Read the model definition and answer for the solid it produces. Units are mm, in the model's axes. A direction names the side the tool comes from. Give positions to 0.01 mm unless a question says otherwise; leave off trailing zeros. Order: outer loops, then holes, each group sorted by start corner. A loop starts at its lowest first (then second) coordinate and runs counter-clockwise, first axis right, second up.
```python
from build123d import *

# Parameters (mm, degrees)
BOSS_EXTRUDE1_DEPTH = 6.35
CUT_EXTRUDE3_DEPTH  = 4.953
SKETCH7_W           = 6.35
SKETCH7_H           = 6.35
CUT_EXTRUDE5_DEPTH  = 2.159
SKETCH9_R           = 3.175
BOSS_EXTRUDE4_DEPTH = 26.035
CUT_EXTRUDE6_REACH  = 34.945
SKETCH10_W          = 1.886216022
SKETCH10_H          = 12.7
FILLET1_R           = 1.27


with BuildPart() as part:
    # Sketch1 → Boss-Extrude1 (new body)
    with BuildSketch(Plane(origin=(0, 0, 0), x_dir=(1, 0, 0), z_dir=(0, 1, 0))):
        with BuildLine():
            Line((0.583306021, 0), (5.131693979, 0))
            ThreePointArc((5.131693979, 0), (5.661763503, 0.115908886), (6.095077487, 0.442478269))
            Line((6.095077487, 0.442478269), (9.2075, 4.953))
            Line((9.2075, 4.953), (6.0325, 4.953))
            Line((6.0325, 4.953), (6.0325, 7.112))
            Line((6.0325, 7.112), (-0.3175, 7.112))
            Line((-0.3175, 7.112), (-0.3175, 4.953))
            Line((-0.3175, 4.953), (-3.4925, 4.953))
            Line((-3.4925, 4.953), (-0.380077487, 0.442478269))
            ThreePointArc((-0.380077487, 0.442478269), (0.053236497, 0.115908886), (0.583306021, 0))
        make_face()
    extrude(amount=BOSS_EXTRUDE1_DEPTH)

    # Sketch5 → Cut-Extrude3 (cut)
    with BuildSketch(Plane.XY):
        with BuildLine():
            Line((-3.4925, 3.175), (-3.4925, 6.35))
            Line((-3.4925, 6.35), (-0.380077487, 6.35))
            add(Edge.make_bspline(
                [(-3.4925, 3.175), (-2.286021044, 5.595085513), (-0.380077487, 6.35)],
                knots=[0, 0, 0, 0.524463315, 0.524463315, 0.524463315], degree=2))
        make_face()
        with BuildLine():
            Line((6.095077487, 0), (9.2075, 0))
            Line((9.2075, 0), (9.2075, 3.175))
            add(Edge.make_bspline(
                [(9.2075, 3.175), (8.001021011, 0.754914499), (6.095077487, 0)],
                knots=[0, 0, 0, 0.524463308, 0.524463308, 0.524463308], degree=2))
        make_face()
        with BuildLine():
            Line((9.2075, 6.35), (9.2075, 5.2705))
            ThreePointArc((9.2075, 5.2705), (8.848057048, 5.990557048), (8.128, 6.35))
            Line((8.128, 6.35), (9.2075, 6.35))
        make_face()
        with BuildLine():
            Line((-3.4925, 0), (-2.413, 0))
            ThreePointArc((-2.413, 0), (-3.133057048, 0.359442952), (-3.4925, 1.0795))
            Line((-3.4925, 1.0795), (-3.4925, 0))
        make_face()
    extrude(amount=-CUT_EXTRUDE3_DEPTH, mode=Mode.SUBTRACT)

    # Sketch7 → Cut-Extrude5 (cut)
    with BuildSketch(Plane(origin=(0, 0, -7.112), x_dir=(-1, 0, 0), z_dir=(0, 0, -1))):
        with Locations((-2.8575, 3.175)):
            Rectangle(SKETCH7_W, SKETCH7_H)
    extrude(amount=-CUT_EXTRUDE5_DEPTH, mode=Mode.SUBTRACT)

    # Sketch9 → Boss-Extrude4 (add)
    with BuildSketch(Plane(origin=(0, 0, -4.953), x_dir=(-1, 0, 0), z_dir=(0, 0, -1))):
        with Locations(Location((-2.8575, 3.175, 0), (0, 0, 270))):
            Circle(SKETCH9_R)
    extrude(amount=BOSS_EXTRUDE4_DEPTH)

    # Cut-Extrude6: up to this face of the body (flat: up to its plane)
    cut_extrude6_end = Plane(part.part.faces().sort_by_distance((2.192673253, 0, -2.628972318))[0])
    # Sketch10 → Cut-Extrude6 (cut, up to the picked face)
    with BuildSketch(Plane(origin=(0, 6.35, 0), x_dir=(1, 0, 0), z_dir=(0, 1, 0)), mode=Mode.PRIVATE) as cut_extrude6_sk1:
        with Locations((2.8575, 6.35)):
            Rectangle(SKETCH10_W, SKETCH10_H)
    cut_extrude6_tool1 = split(extrude(cut_extrude6_sk1.sketch, amount=-CUT_EXTRUDE6_REACH, mode=Mode.PRIVATE), bisect_by=cut_extrude6_end, keep=Keep.BOTH, mode=Mode.PRIVATE)
    add(cut_extrude6_tool1.solids().sort_by(Axis((2.8575, 6.35, -6.35), (0, -1, 0)))[0], mode=Mode.SUBTRACT)

    # Fillet1
    # the kernel refuses this fillet: 1.27 mm, written as the material it adds along each edge
    with BuildSketch(Plane(origin=(1.914391989, 9.381694622, -12.7), x_dir=(1, 0, 0), z_dir=(0, -1, 0))) as fillet1_piece_1_section:
        with BuildLine():
            CenterArc((FILLET1_R, FILLET1_R), FILLET1_R, 180, 90)
            Line((0, FILLET1_R), (0, 0))
            Line((0, 0), (FILLET1_R, 0))
        make_face()
    fillet1_piece_1 = extrude(amount=12.413389243, mode=Mode.PRIVATE)
    fillet1_piece_1 = fillet1_piece_1 & Plane(origin=(2.8575, 3.175, -12.415110082), x_dir=(0, -1, 0), z_dir=(0, 0, 1)) * Cylinder(3.175, 30, mode=Mode.PRIVATE)
    add(fillet1_piece_1)
    with BuildSketch(Plane(origin=(3.800608011, 9.381694622, -12.7), x_dir=(0, 0, 1), z_dir=(0, -1, 0))) as fillet1_piece_2_section:
        with BuildLine():
            CenterArc((FILLET1_R, FILLET1_R), FILLET1_R, 180, 90)
            Line((0, FILLET1_R), (0, 0))
            Line((0, 0), (FILLET1_R, 0))
        make_face()
    fillet1_piece_2 = extrude(amount=12.413389243, mode=Mode.PRIVATE)
    fillet1_piece_2 = fillet1_piece_2 & Plane(origin=(2.8575, 3.175, -12.415110016), x_dir=(0, -1, 0), z_dir=(0, 0, 1)) * Cylinder(3.175, 30, mode=Mode.PRIVATE)
    add(fillet1_piece_2)


solid = part.part
```
1) The part is cut by section A-A on x = 4.25. Determine the outline of the cut face in (y, z).
Final values:
outline: (0, -4.95) - (0.32, -4.95) - (0.32, -30.99) - (6.03, -30.99) - (6.03, -4.95) - (6.35, -4.95) - (6.35, 0) - (0, 0) - close
2) For a pull along X with two mould halves and no side action, classify faces 4 (the face through (5.65, 3.13, -0.11)), 5 (the face through (3.53, 3.219, -12.213)), 6 (the face through (-1, 3, -4.953)) as released by +X, released by -X, zero draft, split by the parting line, or undercut.
Final values:
face 4: released by +X
face 5: undercut
face 6: zero draft
3) Given pin 1 (2 mm diameter, centred on y = 2, z = -5, fed in from +X); pin 2 (1 mm diameter, centred on x = 5, z = -23, fed in from -Y); pin 3 (2.5 mm diameter, centred on x = 7.5, y = 3.5, fed in from -Z), each flat-ended and moving along its own axis, determine where each tip first touches the part or whether it passes through.
Final values:
pin 1: stops at x = 9.12
pin 2: stops at y = 0.46
pin 3: stops at z = -4.95
4) The part is cut by section D-D on x = 0. Determine the outline of the cut face in (y, z), and give its area (3 significant figures).
Final values:
outline: (0, -4.95) - (1.79, -4.95) - (1.79, -30.99) - (4.56, -30.99) - (4.56, -4.95) - (6.35, -4.95) - (6.35, -0.14) - (0, -0.14) - close
area: 103 mm2
5) Consider L1, parallel to X at y = 3, z = -6.5; L2, parallel to X at y = 2, z = -1; L3, parallel to X at y = 3, z = -22. Determine where each line is inside the solid, lowest interval first.
Final values:
L1: x = -0.31 to 1.91, 3.8 to 6.03
L2: x = -0.76 to 1.91, 3.8 to 6.48
L3: x = -0.31 to 6.03
6) A tool of negligible diameter and unlimited length cuts with its end or side. For faces 1 (the face through (5, 6.35, -3)), 2 (the face through (1.914, 3, -6)), 3 (the face through (7, 4, -4.953)), from which of +Z, -Z, +X, -X, +Y, -Y can it reach the whole face along a straight path? Write none if from no direction.
Final values:
face 1: +Z, -Z, +X, -X, +Y
face 2: +Z, +Y, -Y
face 3: -Z, +X
